Verification items for the finished model (mm, model axes). Face numbers are marked on the shaded views. A direction names the side the tool comes from. Round coordinates to 2 decimals unless told otherwise and drop trailing zeros. Order: outer loops, then holes, each group sorted by start corner. A loop starts at its lowest first (then second) coordinate and runs counter-clockwise, first axis right, second up. Notation, with made-up numbers: M -4,1 L 28,1 A18 ccw 28,30 Z; hole C 50.25,13.5 d8. An arc over 180 degrees is marked long. Use one line per item in the form item = value. Start each with the question number.
Item 1: Cross-section at A-A on z = 6.25. Enter the section's corners in (x, y), then the cut area to 3 significant figures.
Item 2: Release check for a two-part mould opening along Y. For the marked faces 1, 2 and 3 record: +Y half, -Y half, draft (parallel to the pull), parting line (faces both ways), or undercut.
Item 3: Thickness scan on probe 1 along Y at (x, z) = (4.5, 5.25); probe 2 along X at (y, z) = (8.75, -0.5); probe 3 along Z at (x, y) = (4.75, 3). Record the ranges inside material, lowest first. Write a range as [from, to].
Item 4: Cross-section at C-C on x = 1. Enter the section's corners in (y, z), then the cut area to 4 significant figures.
Item 5: Tool access check on the marked faces 4 and 5. Record the directions out of +Z, -Z, +X, -X, +Y, -Y that give a thin tool (end or side, any length) a straight path to the whole face; none if there is none.
Item 6: Cross-section at B-B on y = 11.75. Enter the section's corners in (x, z).
Item 7: Go/stop test with flat-tipped pins: pin 1 Ø2 at (x, y) = (3.5, 3.5) entering from +Z; pin 2 Ø5 at (x, z) = (-1.5, 3.5) entering from -Y. Record where each tip stops, or that it passes through.
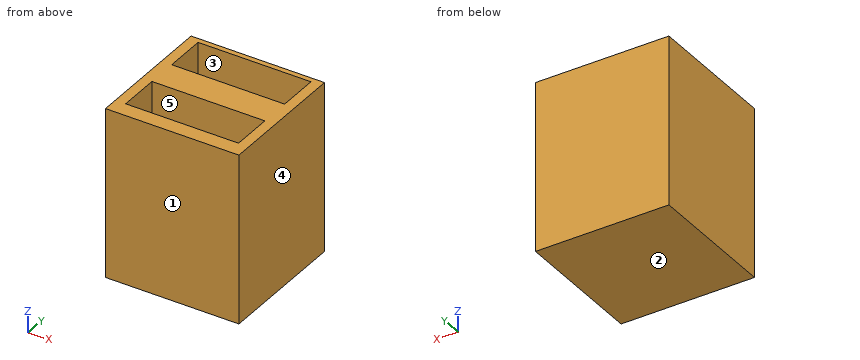
Autodesk Inventor part; units mm, degrees
ref_plane "YZ Plane" through (0, 0, 0) normal (1, 0, 0) x (0, 1, 0)
ref_plane "XZ Plane" through (0, 0, 0) normal (0, 1, 0) x (-1, 0, 0)
ref_plane "XY Plane" through (0, 0, 0) normal (0, 0, 1) x (1, 0, 0)
sketch "Sketch1" plane through (0, 0, 0) normal (0, 1, 0) x (-1, 0, 0)
  line L0 (-6.5, 8.25) -> (6.5, 8.25)
  line L1 (6.5, 8.25) -> (6.5, -8.25)
  line L2 (6.5, -8.25) -> (-6.5, -8.25)
  line L3 (-6.5, -8.25) -> (-6.5, 8.25)
  line L4 (-6.5, 8.25) -> (6.5, -8.25) construction
  line L5 (6.5, 8.25) -> (-6.5, -8.25) construction
  point P0 (0, 0)
  dimension "d0" = 13
  dimension "d1" = 16.5
extrude "Extrusion1" add sketch "Sketch1" along normal blind 13
sketch "Sketch2" plane through (-6.5, 0, 8.25) normal (0, 0, 1) x (1, 0, 0)
  line L0 (1, 8.5) -> (12, 8.5)
  line L1 (12, 8.5) -> (12, 12.5)
  line L2 (12, 12.5) -> (1, 12.5)
  line L3 (1, 12.5) -> (1, 8.5)
  line L4 (0, 13) -> (13, 13)
  line L5 (0, 0) -> (0, 13)
  line L6 (1, 5.5) -> (12, 5.5)
  line L7 (12, 5.5) -> (12, 1.5)
  line L8 (12, 1.5) -> (1, 1.5)
  line L9 (1, 1.5) -> (1, 5.5)
  point P0 (6.5, 0)
  dimension "d4" = 11
  dimension "d5" = 4
  dimension "d6" = 0.5
  dimension "d7" = 1
  dimension "d8" = 11
  dimension "d9" = 4
  dimension "d10" = 3
  dimension "d11" = 1
extrude "Extrusion2" cut sketch "Sketch2" against normal blind 13
properties part number "USB"
Output values:
q1.outline = M -6.5,0 L 6.5,0 L 6.5,13 L -6.5,13 Z; hole M -5.5,1.5 L 5.5,1.5 L 5.5,5.5 L -5.5,5.5 Z; hole M -5.5,8.5 L 5.5,8.5 L 5.5,12.5 L -5.5,12.5 Z
q1.area = 81.0 mm2
q2.face_1 = -Y half
q2.face_2 = draft
q2.face_3 = undercut
q3.probe_1 = [0, 1.5], [5.5, 8.5], [12.5, 13]
q3.probe_2 = [-6.5, -5.5], [5.5, 6.5]
q3.probe_3 = [-8.25, -4.75]
q4.outline = M 0,-8.25 L 13,-8.25 L 13,8.25 L 12.5,8.25 L 12.5,-4.75 L 8.5,-4.75 L 8.5,8.25 L 5.5,8.25 L 5.5,-4.75 L 1.5,-4.75 L 1.5,8.25 L 0,8.25 Z
q4.area = 110.5 mm2
q5.face_4 = +Z, -Z, +X, +Y, -Y
q5.face_5 = +Z
q6.outline = M -6.5,-8.25 L 6.5,-8.25 L 6.5,8.25 L 5.5,8.25 L 5.5,-4.75 L -5.5,-4.75 L -5.5,8.25 L -6.5,8.25 Z
q7.pin_1 = -4.75
q7.pin_2 = 0
